Source: CAD feature listing. Evaluate the final solid. Frame: model axes, mm. Face numbers are marked on the shaded views. A direction names the side the tool comes from. Round coordinates to 2 decimals unless told otherwise and drop trailing zeros. Loops run counter-clockwise (first coordinate to the right, second up) from the corner with the lowest first, then second, coordinate; pieces in that order, holes last. Notation, with made-up numbers: (-20, 67) - (-1, 67) arc R25 ccw to (-1, 88) - close; hole circle Ø1 at (-13, 67). An arc over 180 degrees is marked (long way). Write item = value, one per line. Start each with the question number.
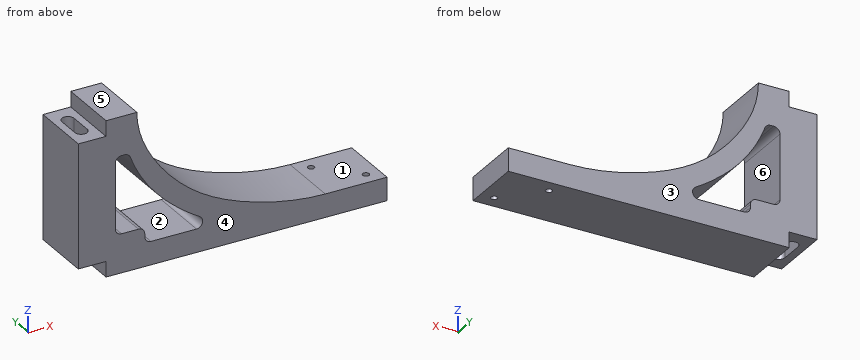
from build123d import *

# Parameters (mm, degrees)
BOSS_EXTRUDE1_DEPTH = 20
SKETCH3_R           = 1.05
CUT_EXTRUDE1_DEPTH  = 20
CUT_EXTRUDE2_DEPTH  = 40


with BuildPart() as part:
    # Sketch2 → Boss-Extrude1 (new body)
    with BuildSketch(Plane(origin=(0, 0, 0), x_dir=(1, 0, 0), z_dir=(0, 1, 0))):
        with BuildLine():
            Line((-28.658256337, 0.746179815), (-28.658256337, -39.253820185))
            Line((-28.658256337, -39.253820185), (-19.658256337, -39.253820185))
            Line((-19.658256337, -39.253820185), (-19.658256337, -44.253820185))
            Line((-19.658256337, -44.253820185), (-9.658256337, -44.253820185))
            add(Edge.make_bspline(
                [(51.341743663, -1.753820185), (43.95022076, -1.753820185), (29.066773176, -4.285907938), (9.29440035, -12.327662678), (-4.675837532, -26.625913431), (-9.658256337, -37.88850288), (-9.658256337, -44.253820185)],
                knots=[0, 0, 0, 0, 0.278287614, 0.548949831, 0.780652353, 1, 1, 1, 1], degree=3))
            Line((51.341743663, -1.753820185), (71.341743663, -1.753820185))
            Line((71.341743663, -1.753820185), (71.341743663, 5.746179815))
            Line((71.341743663, 5.746179815), (-19.658256337, 5.746179815))
            Line((-19.658256337, 5.746179815), (-19.658256337, 0.746179815))
            Line((-19.658256337, 0.746179815), (-28.658256337, 0.746179815))
        make_face()
        with BuildLine():
            Line((-16.658256337, -8.753820185), (-16.658256337, -29.753820185))
            ThreePointArc((-16.658256337, -29.753820185), (-16.072469899, -31.168033747), (-14.658256337, -31.753820185))
            Line((-14.658256337, -31.753820185), (-13.658256337, -31.753820185))
            ThreePointArc((-13.658256337, -31.753820185), (-12.516927691, -31.396187051), (-11.783775986, -30.451189107))
            add(Edge.make_bspline(
                [(-11.783775986, -30.451189107), (-11.274185157, -29.081443531), (-9.924306316, -25.969887858), (-6.252653639, -19.752734333), (0.001148732, -12.823138849), (6.367068894, -8.07935758), (10.008653919, -5.860320829), (10.658890446, -5.478714099)],
                knots=[0.457049826, 0.457049826, 0.457049826, 0.457049826, 0.498595934, 0.553238181, 0.662522676, 0.771807171, 0.79534653, 0.79534653, 0.79534653, 0.79534653], degree=3))
            ThreePointArc((10.658890446, -5.478714099), (11.576593959, -3.229314622), (9.646595536, -1.753820185))
            Line((9.646595536, -1.753820185), (-5.120566965, -1.753820185))
            ThreePointArc((-5.120566965, -1.753820185), (-6.534780528, -2.339606623), (-7.120566965, -3.753820185))
            Line((-7.120566965, -3.753820185), (-7.120566965, -4.753820185))
            ThreePointArc((-7.120566965, -4.753820185), (-7.706353403, -6.168033747), (-9.120566965, -6.753820185))
            Line((-9.120566965, -6.753820185), (-14.658256337, -6.753820185))
            ThreePointArc((-14.658256337, -6.753820185), (-16.072469899, -7.339606623), (-16.658256337, -8.753820185))
        make_face(mode=Mode.SUBTRACT)
    extrude(amount=BOSS_EXTRUDE1_DEPTH)

    # Sketch3 → Cut-Extrude1 (cut)
    with BuildSketch(Plane(origin=(0, 0, -5.746179815), x_dir=(-1, 0, 0), z_dir=(0, 0, -1))):
        with Locations((-55.684889413, 15.656854249)):
            Circle(SKETCH3_R)
        with Locations((-66.998597912, 4.343145751)):
            Circle(SKETCH3_R)
    extrude(amount=-CUT_EXTRUDE1_DEPTH, mode=Mode.SUBTRACT)

    # Sketch4 → Cut-Extrude2 (cut)
    with BuildSketch(Plane(origin=(0, 0, -0.746179815), x_dir=(-1, 0, 0), z_dir=(0, 0, -1))):
        with BuildLine():
            Line((22.158256337, 6.25), (22.158256337, 13.75))
            ThreePointArc((22.158256337, 13.75), (24.158256337, 15.75), (26.158256337, 13.75))
            Line((26.158256337, 13.75), (26.158256337, 6.25))
            ThreePointArc((26.158256337, 6.25), (24.158256337, 4.25), (22.158256337, 6.25))
        make_face()
    extrude(amount=-CUT_EXTRUDE2_DEPTH, mode=Mode.SUBTRACT)


solid = part.part
(1) Cut plane A-A (y = 12.25). State how many separate pieces and enclosed holes the cut face has, and give its area (3 significant figures).
(2) Access query for the marked faces 1, 2 and 3. Directions: +Z, -Z, +X, -X, +Y, -Y. A direction counts if a zero-diameter tool reaches every point of the face in a straight line with its end or side. Return the directions, or none.
(3) Mould query, pull axis Z, two halves, no side actions, for the marked faces 4, 5 and 6. Classes: +Z half, -Z half, draft (parallel to the pull), parting line (faces both ways), or undercut.
(4) Cut plane C-C (x = 62.5). Output: boundary loops of the cut face in (y, z).
(5) Pin query (flat end, axial travel): P1, Ø2.5, axis at x = -22.5, y = 13, coming from the -Z side; P2, Ø1.9, axis at x = 67, y = 4.34, coming from the -Z side; P3, Ø4, axis at x = 40.5, y = 11.5, coming from the +Z side; P4, Ø8, axis at x = 10, y = 11.5, coming from the +Z side. Return the tip coordinate at first contact, or that it passes through.
(6) Material intervals for line 1 along Z through (x, y) = (60, 18); line 2 along X through (y, z) = (15.5, 16.5); line 3 along X through (y, z) = (11, 12.5), sorted ascending. Write a range as from..to.
Solution:
q1.separate_pieces = 2
q1.enclosed_holes = 1
q1.area = 1,500 mm^2
q2.face_1 = +Z, +X, +Y, -Y
q2.face_2 = +Y, -Y
q2.face_3 = +Z, -Z, +X, -X, +Y
q3.face_4 = draft
q3.face_5 = +Z half
q3.face_6 = undercut
q4.outline = (0, -5.75) - (20, -5.75) - (20, 1.75) - (0, 1.75) - close
q5.P1 = -0.75
q5.P2 = through
q5.P3 = 2.94
q5.P4 = 16.53
q6.line_1 = -5.75..1.75
q6.line_2 = -28.66..-25.13, -23.19..-16.66, -3.18..6.04
q6.line_3 = -28.66..-26.16, -22.16..-16.66, 0.9..11.65
